```python
from build123d import *

# Parameters (mm, degrees)
F1_DEPTH             = 6.35
F3_DEPTH             = 19.05
F4_DEPTH             = 6.351
F5_SIZE              = 1.27
F6_SIZE              = 1.27
F9_D                 = 3.81
F9_CBORE_D           = 6.35
F9_CBORE_DEPTH       = 5.08
F9_ON_F8_D           = 3.81
F9_ON_F8_CBORE_D     = 6.35
F9_ON_F8_CBORE_DEPTH = 5.08


with BuildPart() as f1:
    # F0 (on Front) → F1 (new body)
    with BuildSketch(Plane.XZ):
        with BuildLine():
            ThreePointArc((31.75, 12.7), (29.8901280605, 17.1901280605), (25.4, 19.05))
            Line((25.4, 19.05), (-25.4, 19.05))
            ThreePointArc((-25.4, 19.05), (-29.8901280605, 17.1901280605), (-31.75, 12.7))
            Line((-31.75, 12.7), (-31.75, -19.05))
            Line((-31.75, -19.05), (31.75, -19.05))
            Line((31.75, -19.05), (31.75, 12.7))
        make_face()
    extrude(amount=F1_DEPTH)

    # F2 (on face) → F3 (join)
    with BuildSketch(Plane.XZ.offset(6.35)):
        with BuildLine():
            Line((19.05, -19.05), (25.4, -19.05))
            Line((25.4, -19.05), (25.4, 0))
            Line((25.4, 0), (22.225, 0))
            ThreePointArc((22.225, 0), (17.7348719395, 1.8598719395), (15.875, 6.35))
            Line((15.875, 6.35), (15.875, 19.05))
            Line((15.875, 19.05), (12.7, 19.05))
            ThreePointArc((12.7, 19.05), (0, 6.35), (-12.7, 19.05))
            Line((-12.7, 19.05), (-15.875, 19.05))
            Line((-15.875, 19.05), (-15.875, 6.35))
            ThreePointArc((-15.875, 6.35), (-17.7348719395, 1.8598719395), (-22.225, 0))
            Line((-22.225, 0), (-25.4, 0))
            Line((-25.4, 0), (-25.4, -19.05))
            Line((-25.4, -19.05), (-19.05, -19.05))
            Line((-19.05, -19.05), (-19.05, -8.89))
            Line((-19.05, -8.89), (19.05, -8.89))
            Line((19.05, -8.89), (19.05, -19.05))
        make_face()
    extrude(amount=F3_DEPTH)

    # F4 (cut, through all): a face of the model
    f4_faces = [f1.faces().sort_by_distance(p)[0] for p in [
        (0, -6.35, 13.659952594),
    ]]
    extrude(f4_faces, amount=-F4_DEPTH, mode=Mode.SUBTRACT)

    # F5
    f5_edges = [f1.edges().sort_by_distance(p)[0] for p in [
        (0, -25.4, -8.89),
        (-19.05, -25.4, -13.97),
        (19.05, -25.4, -13.97),
    ]]
    chamfer(f5_edges, length=F5_SIZE)

    # F6
    f6_edges = [f1.edges().sort_by_distance(p)[0] for p in [
        (0, -25.4, 6.35),
    ]]
    chamfer(f6_edges, length=F6_SIZE)

    # F9 (through all)
    with Locations(Plane.XZ.offset(6.35)):
        with Locations((-25.4, 12.7)):
            CounterBoreHole(F9_D / 2, F9_CBORE_D / 2, F9_CBORE_DEPTH)

    # F9 on F8 (through all)
    with Locations(Plane.XZ.offset(6.35)):
        with Locations((25.4, 12.7)):
            CounterBoreHole(F9_ON_F8_D / 2, F9_ON_F8_CBORE_D / 2, F9_ON_F8_CBORE_DEPTH)


solid = f1.part
```
Read the model definition and answer for the solid it produces. Units are mm, in the model's axes. A direction names the side the tool comes from. Give positions to 0.01 mm unless a question says otherwise; leave off trailing zeros. Write each loop counter-clockwise with the first axis right and the second up, starting at its lowest first coordinate (ties: lowest second). Pieces come first, ordered by that corner, then holes. Notation, with made-up numbers: (29.25, 35.5) - (69.25, 35.5) arc R18 ccw to (69.25, 45.5) - close; hole circle Ø9 at (18, -39). An arc over 180 degrees is marked (long way). Write item = value, one per line. Start each with the question number.
Item 1: Find the intervals of material crossed by probe 1 along Z at (x, y) = (25.4, -5.25) (3 decimals); probe 2 along Z at (x, y) = (25.4, -0.9) (3 decimals); probe 3 along Y at (x, z) = (-28, 1.5), in increasing order. Write a range as [from, to].
Item 2: The mould has two halves that part along Z. Classify faces 5 (the flat face through (-24, -16, 0)), 6 (the cylindrical face through (-23.497, -0.626, 12.784)), 7 (the flat face through (-26, -6.35, 5)): +Z half, -Z half, draft (parallel to the pull), parting line (faces both ways), or undercut.
Item 3: Each of these flat-tipped pins is pushed along its axis until it touches: P1, Ø1.6, axis at x = 24, y = -16, coming from the +Z side; P2, Ø8, axis at x = 2.5, y = -19, coming from the -Z side; P3, Ø15, axis at y = -11.5, z = -9.5, coming from the +X side; P4, Ø5.5, axis at y = -16.5, z = -8.5, coming from the -X side. Where does it stop, or does it pass through?
Item 4: Find section D-D (x = 17). Give the vertices of the cut face in (y, z), then the cut area to 3 significant figures.
Item 5: A tool of negligible diameter and unlimited length cuts with its end or side. For faces 1 (the flat face through (-19.68, -24.76, -13.42)), 2 (the flat face through (27, -1.27, 11)), 3 (the flat face through (25.4, -16, -10)), 4 (the cylindrical face through (-17.686, -15.742, 1.91)), from which of +Z, -Z, +X, -X, +Y, -Y can it reach the whole face along a straight path? Write none if from no direction.
Item 6: Find section B-B (y = -7). Give the vertices of the cut face in (x, z) (3 decimals).
Item 7: Find section A-A (z = -2). Give the vertices of the cut face in (x, y), then the cut area to 3 significant figures.
Item 8: Find section C-C (x = 0). Give the vertices of the cut face in (y, z), then the cut area to 3 significant figures.
Response:
q1.probe_1 = [-19.05, 9.525], [15.875, 19.05]
q1.probe_2 = [-19.05, 10.795], [14.605, 19.05]
q1.probe_3 = [-6.35, 0]
q2.face_5 = +Z half
q2.face_6 = undercut
q2.face_7 = draft
q3.P1 = 0
q3.P2 = -8.89
q3.P3 = 31.75
q3.P4 = -25.4
q4.outline = (-25.4, -7.62) - (-24.13, -8.89) - (-6.35, -8.89) - (-6.35, -19.05) - (0, -19.05) - (0, 19.05) - (-6.35, 19.05) - (-6.35, 2.74) - (-25.4, 2.74) - close
q4.area = 463 mm²
q5.face_1 = -Z, -Y
q5.face_2 = -Y
q5.face_3 = +Z, -Z, +X, -Y
q5.face_4 = +Z, -X, -Y
q6.outline = (-25.4, -19.05) - (-19.05, -19.05) - (-19.05, -8.89) - (19.05, -8.89) - (19.05, -19.05) - (25.4, -19.05) - (25.4, 0) - (22.225, 0) arc R6.35 cw to (15.875, 6.35) - (15.875, 19.05) - (12.7, 19.05) arc R12.7 cw to (-12.7, 19.05) - (-15.875, 19.05) - (-15.875, 6.35) arc R6.35 cw to (-22.225, 0) - (-25.4, 0) - close
q7.outline = (-31.75, -6.35) - (-25.4, -6.35) - (-25.4, -25.4) - (25.4, -25.4) - (25.4, -6.35) - (31.75, -6.35) - (31.75, 0) - (-31.75, 0) - close
q7.area = 1,370 mm²
q8.outline = (-25.4, -7.62) - (-24.13, -8.89) - (-6.35, -8.89) - (-6.35, -19.05) - (0, -19.05) - (0, 6.35) - (-24.13, 6.35) - (-25.4, 5.08) - close
q8.area = 450 mm²
